Geometry: final body of the model. Coordinates: model frame, mm. Face numbers are marked on the shaded views. Round coordinates to 2 decimals unless told otherwise and drop trailing zeros. Write each loop counter-clockwise with the first axis right and the second up, starting at its lowest first coordinate (ties: lowest second). Pieces come first, ordered by that corner, then holes. Notation, with made-up numbers: (-30.5, 17) -> (-22.5, 17) arc R24 cw to (-22.5, 43) -> close; hole circle Ø2 at (77.5, -11). An arc over 180 degrees is marked (long way). One line per item, written item: value. Start each with the question number.
from build123d import *

# Parameters (mm, degrees)
SKETCH2_W                                            = 70
SKETCH2_H                                            = 50
BOSS_EXTRUDE1_DEPTH                                  = 10
SKETCH3_R                                            = 4
CUT_EXTRUDE1_DEPTH                                   = 11
SKETCH4_R                                            = 1.8
CUT_EXTRUDE2_DEPTH                                   = 11
SKETCH5_R                                            = 10
CUT_EXTRUDE3_DEPTH                                   = 11
CSK_FOR_M3_SOCKET_COUNTERSUNK_HEAD_SCREW_D           = 3.4
CSK_FOR_M3_SOCKET_COUNTERSUNK_HEAD_SCREW_CSINK_D     = 6.94
CSK_FOR_M3_SOCKET_COUNTERSUNK_HEAD_SCREW_CSINK_ANGLE = 90


with BuildPart() as part:
    # Sketch2 → Boss-Extrude1 (new body)
    with BuildSketch(Plane(origin=(0, 0, 0), x_dir=(1, 0, 0), z_dir=(0, 1, 0))):
        Rectangle(SKETCH2_W, SKETCH2_H)
    extrude(amount=BOSS_EXTRUDE1_DEPTH)

    # Sketch3 → Cut-Extrude1 (cut, through all)
    with BuildSketch(Plane(origin=(0, 10, 0), x_dir=(1, 0, 0), z_dir=(0, 1, 0))):
        with Locations((-25, -15)):
            Circle(SKETCH3_R)
        with Locations((25, -15)):
            Circle(SKETCH3_R)
    extrude(amount=-CUT_EXTRUDE1_DEPTH, mode=Mode.SUBTRACT)

    # Sketch4 → Cut-Extrude2 (cut, through all)
    with BuildSketch(Plane.XZ):
        with Locations((-15.5, 19.5)):
            Circle(SKETCH4_R)
        with Locations((-15.5, -11.5)):
            Circle(SKETCH4_R)
        with Locations((15.5, -11.5)):
            Circle(SKETCH4_R)
        with Locations((15.5, 19.5)):
            Circle(SKETCH4_R)
    extrude(amount=-CUT_EXTRUDE2_DEPTH, mode=Mode.SUBTRACT)

    # Sketch5 → Cut-Extrude3 (cut, through all)
    with BuildSketch(Plane.XZ):
        with Locations((0, 4)):
            Circle(SKETCH5_R)
    extrude(amount=-CUT_EXTRUDE3_DEPTH, mode=Mode.SUBTRACT)

    # CSK for M3 socket countersunk head screw (through all)
    with Locations(Plane.XZ):
        with Locations((-15.5, 19.5), (15.5, 19.5), (15.5, -11.5), (-15.5, -11.5)):
            CounterSinkHole(CSK_FOR_M3_SOCKET_COUNTERSUNK_HEAD_SCREW_D / 2, CSK_FOR_M3_SOCKET_COUNTERSUNK_HEAD_SCREW_CSINK_D / 2, counter_sink_angle=CSK_FOR_M3_SOCKET_COUNTERSUNK_HEAD_SCREW_CSINK_ANGLE)


solid = part.part
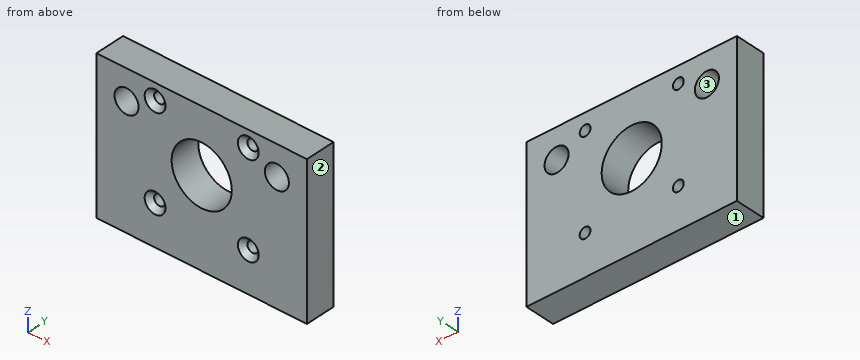
(1) Section query A-A (z = -11.5). Output: boundary loops of the cut face in (x, y).
(2) Section query D-D (z = 4). Output: boundary loops of the cut face in (x, y).
(3) Pull-direction query (X, two-part tool) for the marked faces 1, 2 and 3; classes: pulls with the +X half, pulls with the -X half, needs draft (parallel to the pull), parting line crosses it, or undercut.
(4) Line query: probe 1 along X at (y, z) = (5.75, 19.5); probe 2 along Z at (x, y) = (25, 6.25); probe 3 along X at (y, z) = (8.25, 15). Output: solid intervals per line, ascending.
(5) Section query B-B (x = 0). Output: boundary loops of the cut face in (y, z), and give its area (3 significant figures).
(6) Section query C-C (y = 5.5). Output: boundary loops of the cut face in (x, z), and give its area (3 significant figures).
Results list:
1. outline: (-35, 0) -> (-18.97, 0) -> (-17.3, 1.67) -> (-17.3, 10) -> (-35, 10) -> close; (-13.7, 1.67) -> (-12.03, 0) -> (12.03, 0) -> (13.7, 1.67) -> (13.7, 10) -> (-13.7, 10) -> close; (17.3, 1.67) -> (18.97, 0) -> (35, 0) -> (35, 10) -> (17.3, 10) -> close
2. outline: (-35, 0) -> (-10, 0) -> (-10, 10) -> (-35, 10) -> close; (10, 0) -> (35, 0) -> (35, 10) -> (10, 10) -> close
3. face 1: needs draft
3. face 2: pulls with the +X half
3. face 3: undercut
4. probe 1: x = -35 to -17.3, -13.7 to 13.7, 17.3 to 35
4. probe 2: z = -25 to 11, 19 to 25
4. probe 3: x = -35 to -29, -21 to 21, 29 to 35
5. outline: (0, -25) -> (10, -25) -> (10, -6) -> (0, -6) -> close; (0, 14) -> (10, 14) -> (10, 25) -> (0, 25) -> close
5. area: 300 mm^2
6. outline: (-35, -25) -> (35, -25) -> (35, 25) -> (-35, 25) -> close; hole circle Ø8 at (-25, 15); hole circle Ø3.6 at (-15.5, -11.5); hole circle Ø3.6 at (-15.5, 19.5); hole circle Ø20 at (0, 4); hole circle Ø3.6 at (15.5, -11.5); hole circle Ø3.6 at (15.5, 19.5); hole circle Ø8 at (25, 15)
6. area: 3,040 mm^2
